Model file for the job. Use its own axes, mm. A direction names the side the tool comes from. Give positions to 0.01 mm unless a question says otherwise; leave off trailing zeros. Write each loop counter-clockwise with the first axis right and the second up, starting at its lowest first coordinate (ties: lowest second). Pieces come first, ordered by that corner, then holes. Notation, with made-up numbers: (38, 28.5) - (55, 28.5) arc R36 ccw to (55, 63.5) - close; hole circle Ø5 at (73.5, -37). An arc over 180 degrees is marked (long way). Use a Markdown table: item, result. Add a question column.
```python
from build123d import *

# Parameters (mm, degrees)
SKETCH1_R               = 22
BOSS_EXTRUDE1_DEPTH     = 5
SKETCH2_R               = 22
SKETCH2_R_2             = 20
BOSS_EXTRUDE2_DEPTH     = 0.5
BOSS_EXTRUDE4_START     = -15
SKETCH1_2_R             = 22
BOSS_EXTRUDE4_DEPTH     = 15
BOSS_EXTRUDE5_START     = -10.5
SKETCH2_2_R             = 22
SKETCH2_2_R_2           = 20
BOSS_EXTRUDE5_DEPTH     = 10.5
CUT_EXTRUDE1_DEPTH      = 263.162163555
CUT_EXTRUDE1_DEPTH_BACK = 263.162163555
SKETCH6_W               = 10
SKETCH6_H               = 30
CUT_EXTRUDE2_DEPTH      = 10
SKETCH8_R               = 2.5
CUT_EXTRUDE3_DEPTH      = 27
SKETCH9_R               = 1.75
BOSS_EXTRUDE6_DEPTH     = 5


with BuildPart() as part:
    # Sketch1 → Boss-Extrude1 (new body)
    with BuildSketch(Plane.XY):
        with BuildLine():
            Line((-27, -260), (27, -260))
            Line((27, -260), (27, 0))
            ThreePointArc((27, 0), (0, 27), (-27, 0))
            Line((-27, 0), (-27, -260))
        make_face()
        Circle(SKETCH1_R, mode=Mode.SUBTRACT)
    extrude(amount=BOSS_EXTRUDE1_DEPTH)

    # Sketch2 → Boss-Extrude2 (add)
    with BuildSketch(Plane.XY):
        Circle(SKETCH2_R)
        Circle(SKETCH2_R_2, mode=Mode.SUBTRACT)
    extrude(amount=BOSS_EXTRUDE2_DEPTH)

    # Sketch1<2> → Boss-Extrude4 (add)
    with BuildSketch(Plane.XY.offset(BOSS_EXTRUDE4_START)):
        with BuildLine():
            Line((-27, -260), (27, -260))
            Line((27, -260), (27, 0))
            ThreePointArc((27, 0), (0, 27), (-27, 0))
            Line((-27, 0), (-27, -260))
        make_face()
        Circle(SKETCH1_2_R, mode=Mode.SUBTRACT)
    extrude(amount=BOSS_EXTRUDE4_DEPTH)

    # Sketch2<2> → Boss-Extrude5 (add)
    with BuildSketch(Plane.XY.offset(BOSS_EXTRUDE5_START)):
        Circle(SKETCH2_2_R)
        Circle(SKETCH2_2_R_2, mode=Mode.SUBTRACT)
    extrude(amount=BOSS_EXTRUDE5_DEPTH)

    # Sketch6 → Cut-Extrude1 (cut, two sides: drawn at the far end of the back side and taken through both)
    with BuildSketch(Plane.XY.offset(5).offset(-CUT_EXTRUDE1_DEPTH_BACK)):
        with Locations((0, -45)):
            Rectangle(SKETCH6_W, SKETCH6_H)
    extrude(amount=CUT_EXTRUDE1_DEPTH + CUT_EXTRUDE1_DEPTH_BACK, mode=Mode.SUBTRACT)

    # Sketch7 → Cut-Extrude2 (cut)
    with BuildSketch(Plane.XY):
        Polygon((-15, -52.5), (-5, -52.5), (-5, -47.5), (-5, -37.5), (-15, -37.5), align=None)
    extrude(amount=-CUT_EXTRUDE2_DEPTH, mode=Mode.SUBTRACT)

    # Sketch8 → Cut-Extrude3 (cut)
    with BuildSketch(Plane(origin=(0, 0, 0), x_dir=(0, 0, -1), z_dir=(1, 0, 0))):
        with Locations(Location((5, -45, 0), (0, 0, 270))):
            Circle(SKETCH8_R)
    extrude(amount=CUT_EXTRUDE3_DEPTH, mode=Mode.SUBTRACT)

    # Sketch9 → Boss-Extrude6 (add)
    with BuildSketch(Plane(origin=(27, 0, 0), x_dir=(0, 0, -1), z_dir=(1, 0, 0))):
        with Locations(Location((12, -37, 0), (0, 0, 270))):
            Circle(SKETCH9_R)
        with Locations(Location((-1, -58, 0), (0, 0, 270))):
            Circle(SKETCH9_R)
    extrude(amount=BOSS_EXTRUDE6_DEPTH)


solid = part.part
```
(1) Band-saw the part on D-D (y = -8). Write the cut outline in (x, z).
(2) Flat gauge pins, fed straight in: pin 1 (3 mm diameter, centred on y = -136.5, z = 3, fed in from +X); pin 2 (4.5 mm diameter, centred on y = -45, z = -5, fed in from +X); pin 3 (8 mm diameter, centred on x = -12, z = -5, fed in from +Y); pin 4 (12 mm diameter, centred on x = -1.5, y = -20.5, fed in from +Z). Where does each tip first touch, or does it go through?
(3) Two-plate mould, pull along X, no slides. Class faces 5 (the flat face through (10, -18, -10.5)), 6 (the flat face through (-27, -128, -5)), 7 (the cylindrical face through (0.594, 26.993, -5.14)): +X half, -X half, draft (parallel to the pull), parting line (faces both ways), or undercut.
(4) Band-saw the part on B-B (y = -45). Write the cut outline in (x, z), then the cut area to 3 significant figures.
(5) Which spindle directions (+Z, -Z, +X, -X, +Y, -Y) get a long thin tool onto all of the face, cutting with end or side? Do faces 1 (the cylindrical face through (-4.769, -21.477, 2.718)), 2 (the cylindrical face through (-4.769, -21.477, -12.782)), 3 (the flat face through (5, -42, -5)), 4 (the flat face through (-10, -45, 0)). Say none if no direction does.
(6) Band-saw the part on A-A (x = 0). Write the cut outline in (y, z), then the cut area to 3 significant figures.
(7) Probe probe 1 along Y at (x, z) = (0, 2.7); probe 2 along Y at (x, z) = (0, -2); probe 3 along Z at (x, y) = (19.75, -45). List the from-to ranges inside material, lowest first. Write a range as [from, to].
(8) Band-saw the part on C-C (z = -5). Write the cut outline in (x, y).
Model answer:
| question | item | result |
|---|---|---|
| 1 | outline | (-27, -15) - (-20.49, -15) - (-20.49, -10.5) - (-18.33, -10.5) - (-18.33, 0.5) - (-20.49, 0.5) - (-20.49, 5) - (-27, 5) - close; (18.33, -10.5) - (20.49, -10.5) - (20.49, -15) - (27, -15) - (27, 5) - (20.49, 5) - (20.49, 0.5) - (18.33, 0.5) - close |
| 2 | pin 1 | stops at x = 27 |
| 2 | pin 2 | stops at x = -15 |
| 2 | pin 3 | stops at y = 25.79 |
| 2 | pin 4 | stops at z = 5 |
| 3 | face 5 | undercut |
| 3 | face 6 | -X half |
| 3 | face 7 | parting line |
| 4 | outline | (-27, -15) - (-5, -15) - (-5, -10) - (-15, -10) - (-15, 0) - (-5, 0) - (-5, 5) - (-27, 5) - close; (5, -15) - (27, -15) - (27, -7.5) - (5, -7.5) - close; (5, -2.5) - (27, -2.5) - (27, 5) - (5, 5) - close |
| 4 | area | 670 mm^2 |
| 5 | face 1 | +Z |
| 5 | face 2 | -Z |
| 5 | face 3 | +Z, -Z |
| 5 | face 4 | none |
| 6 | outline | (-260, -15) - (-60, -15) - (-60, 5) - (-260, 5) - close; (-30, -15) - (-22, -15) - (-22, -10.5) - (-20, -10.5) - (-20, 0.5) - (-22, 0.5) - (-22, 5) - (-30, 5) - close; (20, -10.5) - (22, -10.5) - (22, -15) - (27, -15) - (27, 5) - (22, 5) - (22, 0.5) - (20, 0.5) - close |
| 6 | area | 4,300 mm^2 |
| 7 | probe 1 | y = [-260, -60], [-30, -22], [22, 27] |
| 7 | probe 2 | y = [-260, -60], [-30, -20], [20, 27] |
| 7 | probe 3 | z = [-15, -7.5], [-2.5, 5] |
| 8 | outline | (-27, -260) - (27, -260) - (27, -47.5) - (5, -47.5) - (5, -60) - (-5, -60) - (-5, -52.5) - (-15, -52.5) - (-15, -37.5) - (-5, -37.5) - (-5, -30) - (5, -30) - (5, -42.5) - (27, -42.5) - (27, 0) arc R27 ccw to (-27, 0) - close; hole circle Ø40 at (0, 0) |
